Autodesk Inventor part; units mm, degrees
ref_plane "YZ Plane" through (0, 0, 0) normal (1, 0, 0) x (0, 1, 0)
ref_plane "XZ Plane" through (0, 0, 0) normal (0, 1, 0) x (-1, 0, 0)
ref_plane "XY Plane" through (0, 0, 0) normal (0, 0, 1) x (1, 0, 0)
sketch "スケッチ1" plane through (0, 0, 0) normal (0, 1, 0) x (-1, 0, 0)
  circle A0 centre (0, 0) radius 3.45
  circle A1 centre (0, 14.1) radius 1.9
  circle A2 centre (0, -14.1) radius 1.9
  line L0 (4.83, 0) -> (-4.83, 0)
  line L1 (1.8885, 14.3089) -> (3.4291, 0.3793)
  line L2 (3.4291, -0.3793) -> (1.8885, -14.3089)
  line L3 (-1.8885, -14.3089) -> (-3.4291, -0.3793)
  line L4 (-3.4291, 0.3793) -> (-1.8885, 14.3089)
  dimension "d0" = 6.9
  dimension "d1" = 3.8
  dimension "d3" = 28.2
extrude "押し出し1" add sketch "スケッチ1" along normal blind 1.4
sketch "スケッチ2" plane through (0, 0, 0) normal (0, -1, 0) x (1, 0, 0)
  circle A0 centre (0, 0) radius 3.45
  arc A1 (3.4291, -0.3793) -> (-3.4291, -0.3793) centre (0, 0) ccw
  point P0 (3.4291, 0.3793)
extrude "押し出し2" add sketch "スケッチ2" along normal blind 2.3
properties part number "Miusei_hone_long"
Design review of the part built by this model. Coordinates are the model's own, in mm. A direction names the side the tool comes from. Give positions to 0.01 mm unless a question says otherwise; leave off trailing zeros. Write each loop counter-clockwise with the first axis right and the second up, starting at its lowest first coordinate (ties: lowest second). Pieces come first, ordered by that corner, then holes. Notation, with made-up numbers: M 6.5,7.25 L 58.5,7.25 A21 cw 58.5,43.25 Z; hole C 29.5,24.5 d8. An arc over 180 degrees is marked long. Answer as a JSON object with one key per item and string values. Group by question number.
1) Tool access review of faces 1 (the face through (-3.433, -0.835, -0.344)), 2 (the face through (0, -2.3, 0)): name each direction out of +Z, -Z, +X, -X, +Y, -Y from which nothing blocks a thin tool from reaching the whole face with its end or side.
2) For line 1 along Y through (x, z) = (1.25, 13); line 2 along Z through (x, y) = (-1.75, -1); line 3 along X through (y, z) = (0.95, -12), list the stretches that pass through material, from the lowest coordinate up.
3) Clearance check with a flat-ended pin moving along its axis: pin 1 Ø1.5 at (x, z) = (2, 12) entering from -Y. State where the tip first meets the part, or that it passes through.
4) We need section B-B (z = -1). Give the boundary of the cut face in (x, y), and give its area (3 significant figures).
5) We need section A-A (x = 0). Give the boundary of the cut face in (y, z).
6) We need section C-C (y = -1.6). Give the boundary of the cut face in (x, z).
7) We need section D-D (z = -6.5). Give the boundary of the cut face in (x, y), and give its area (3 significant figures).
Answer key:
{
 "1": {"face 1": "-Y", "face 2": "+Z, -Z, +X, -X, -Y"},
 "2": {"line 1": "y = 0 to 1.4", "line 2": "z = -2.97 to 2.97", "line 3": "x = -2.14 to 2.14"},
 "3": {"pin 1": "stops at y = 0"},
 "4": {"outline": "M -3.36,0 L -3.3,0 L -3.3,-2.3 L 3.3,-2.3 L 3.3,0 L 3.36,0 L 3.36,1.4 L -3.36,1.4 Z", "area": "24.6 mm²"},
 "5": {"outline": "M -2.3,-3.45 L 0,-3.45 L 0,-16 L 1.4,-16 L 1.4,16 L 0,16 L 0,3.45 L -2.3,3.45 Z"},
 "6": {"outline": "C 0,0 d6.9"},
 "7": {"outline": "M -2.75,0 L 2.75,0 L 2.75,1.4 L -2.75,1.4 Z", "area": "7.71 mm²"}
}
